Drawing for the job (mm, zero at the part's lowest x, y, z). Round coordinates to 2 decimals unless told otherwise and drop trailing zeros. Loops run counter-clockwise (first coordinate to the right, second up) from the corner with the lowest first, then second, coordinate; pieces in that order, holes last. Notation, with made-up numbers: (46, 30) - (58, 30) arc R15 ccw to (58, 51) - close; hole circle Ø9 at (-33, -28.75). An arc over 180 degrees is marked (long way). Put each result on its own line as item: value.
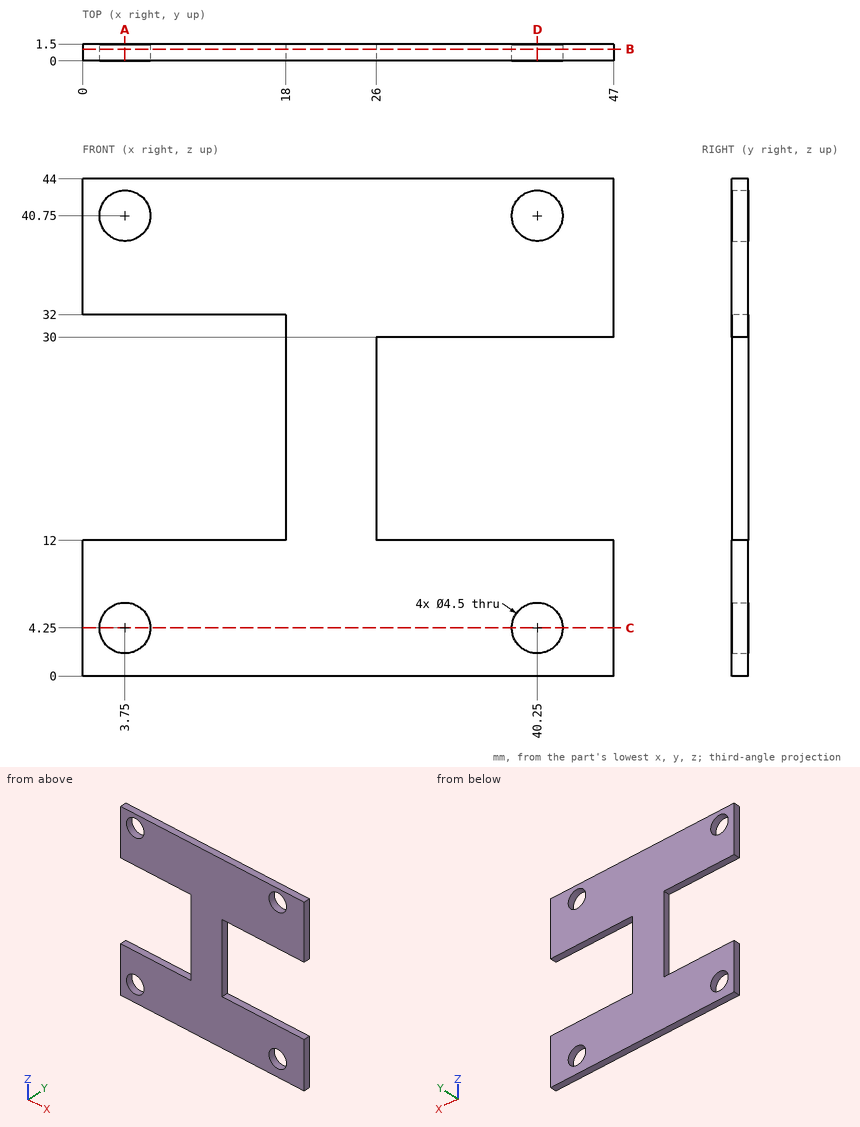
1. Band-saw the part on B-B (y = 1.05). List the corners of the cut face in (x, z), plus the area to 3 significant figures.
A:
outline: (0, 0) - (47, 0) - (47, 12) - (26, 12) - (26, 30) - (47, 30) - (47, 44) - (0, 44) - (0, 32) - (18, 32) - (18, 12) - (0, 12) - close; hole circle Ø4.5 at (3.75, 4.25); hole circle Ø4.5 at (3.75, 40.75); hole circle Ø4.5 at (40.25, 4.25); hole circle Ø4.5 at (40.25, 40.75)
area: 1,270 mm²
2. Band-saw the part on A-A (x = 3.75). List the corners of the cut face in (y, z).
A:
outline: (0, 0) - (1.5, 0) - (1.5, 2) - (0, 2) - close; (0, 6.5) - (1.5, 6.5) - (1.5, 12) - (0, 12) - close; (0, 32) - (1.5, 32) - (1.5, 38.5) - (0, 38.5) - close; (0, 43) - (1.5, 43) - (1.5, 44) - (0, 44) - close
3. Band-saw the part on C-C (z = 4.25). List the corners of the cut face in (x, y), plus the area to 3 significant figures.
A:
outline: (0, 0) - (1.5, 0) - (1.5, 1.5) - (0, 1.5) - close; (6, 0) - (38, 0) - (38, 1.5) - (6, 1.5) - close; (42.5, 0) - (47, 0) - (47, 1.5) - (42.5, 1.5) - close
area: 57.0 mm²
4. Band-saw the part on D-D (x = 40.25). List the corners of the cut face in (y, z), plus the area to 3 significant figures.
A:
outline: (0, 0) - (1.5, 0) - (1.5, 2) - (0, 2) - close; (0, 6.5) - (1.5, 6.5) - (1.5, 12) - (0, 12) - close; (0, 30) - (1.5, 30) - (1.5, 38.5) - (0, 38.5) - close; (0, 43) - (1.5, 43) - (1.5, 44) - (0, 44) - close
area: 25.5 mm²
5. Probe line 1 along Z through (x, y) = (3.75, 0.4); line 2 along Z through (x, y) = (40.25, 0.8); line 3 along X through (y, z) = (0.4, 4.25). List the from-to ranges inside material, lowest first. Write a range as [from, to].
A:
line 1: z = [0, 2], [6.5, 12], [32, 38.5], [43, 44]
line 2: z = [0, 2], [6.5, 12], [30, 38.5], [43, 44]
line 3: x = [0, 1.5], [6, 38], [42.5, 47]
6. Pin check, flat tips, straight feed: P1, Ø7, axis at x = 40.25, z = 40.75, coming from the -Y side; P2, Ø2.5, axis at x = 40.25, z = 4.25, coming from the +Y side. Stop position of each tip, or through.
A:
P1: stops at y = 0
P2: passes through
